Autodesk Inventor part; units mm, degrees
ref_plane "YZ Plane" through (0, 0, 0) normal (1, 0, 0) x (0, 1, 0)
ref_plane "XZ Plane" through (0, 0, 0) normal (0, 1, 0) x (-1, 0, 0)
ref_plane "XY Plane" through (0, 0, 0) normal (0, 0, 1) x (1, 0, 0)
sketch "Sketch1" plane through (0, 0, 0) normal (0, 0, 1) x (1, 0, 0)
  line L0 (-212.725, -63.5) -> (212.725, -63.5)
  line L1 (212.725, -63.5) -> (212.725, 63.5)
  line L2 (212.725, 63.5) -> (-212.725, 63.5)
  line L3 (-212.725, 63.5) -> (-212.725, -63.5)
  line L4 (-212.725, -63.5) -> (212.725, 63.5) construction
  line L5 (212.725, -63.5) -> (-212.725, 63.5) construction
  point P0 (0, 0)
  dimension "d0" = 127
  dimension "d1" = 425.45
extrude "Extrusion1" add sketch "Sketch1" along normal blind 1.5875
sketch "Sketch2" plane through (0, 0, 1.5875) normal (0, 0, 1) x (1, 0, 0)
  line L0 (152.4, -16.2954) -> (-152.4, -16.2954)
  line L1 (-152.4, -16.2954) -> (-152.4, 16.2954)
  line L2 (-152.4, 16.2954) -> (152.4, 16.2954)
  line L3 (152.4, 16.2954) -> (152.4, -16.2954)
  line L4 (152.4, -16.2954) -> (-152.4, 16.2954) construction
  line L5 (-152.4, -16.2954) -> (152.4, 16.2954) construction
  line L6 (-158.4, -5.4991) -> (-146.4, -5.4991)
  line L7 (-146.4, -5.4991) -> (-146.4, 5.4991)
  line L8 (-146.4, 5.4991) -> (-158.4, 5.4991)
  line L9 (-158.4, 5.4991) -> (-158.4, -5.4991)
  line L10 (-158.4, -5.4991) -> (-146.4, 5.4991) construction
  line L11 (-146.4, -5.4991) -> (-158.4, 5.4991) construction
  line L12 (138.9062, -15.4813) -> (165.8937, -15.4813)
  line L13 (165.8937, -15.4813) -> (165.8937, 15.4813)
  line L14 (165.8937, 15.4813) -> (138.9062, 15.4813)
  line L15 (138.9062, 15.4813) -> (138.9062, -15.4813)
  line L16 (138.9062, -15.4813) -> (165.8937, 15.4813) construction
  line L17 (165.8937, -15.4813) -> (138.9062, 15.4813) construction
  point P0 (0, 0)
  point P1 (-137.8966, 0)
  point P2 (-166.9034, 0)
  dimension "d4" = 304.8
  dimension "d5" = 12
  dimension "d6" = 10.9982
  dimension "d9" = 26.9875
  dimension "d10" = 30.9626
extrude "Extrusion2" cut sketch "Sketch2" against normal up to next contours L12 L15 L14 L3 | L3 L14 L13 L12 | L6 L9 L8 L1 | L1 L8 L7 L6
sketch "Sketch3" plane through (0, 0, 1.5875) normal (0, 0, 1) x (1, 0, 0)
  point P0 (0, 0)
hole "Hole1" at (-166.9034, 0, 1.5875) at (-137.8966, 0, 1.5875) direction (0, 0, -1) diameter 3.4036 end through all
sketch "Sketch4" plane through (0, 0, 1.5875) normal (0, 0, 1) x (1, 0, 0)
  point P0 (0, 0)
  point P1 (169.8625, 0)
  point P2 (134.9375, 0)
  point P3 (152.4, 0)
  dimension "d22" = 34.925
  dimension "d23" = 17.4625
  dimension "d24" = 152.4
hole "Hole2" at (134.9375, 0, 1.5875) at (169.8625, 0, 1.5875) direction (0, 0, -1) diameter 3.2766 end through all
properties part number "back"
Part model, mm, in its own coordinate system. Coordinates: 2 decimals unless noted, no trailing zeros. Loops run counter-clockwise (first coordinate to the right, second up) from the corner with the lowest first, then second, coordinate; pieces in that order, holes last. Notation, with made-up numbers: (86, 85) - (112, 85) arc R10 ccw to (112, 92) - close; hole circle Ø5 at (-36, 80.5). An arc over 180 degrees is marked (long way). Write each question's results on one line, items separated by ' | '. Start each with the question number.
Q1. Slice it at C-C on z = 0.5. Give the cut face in (x, y) (1 decimal).
Q2. Probe line 1 along X through (y, z) = (4, 1.15) (3 decimals); line 2 along Y through (x, z) = (158.5, 1.2); line 3 along Y through (x, z) = (-151, 0.8). List the from-to ranges inside material, lowest first.
Q3. Slice it at B-B on y = -10. Give the cut face in (x, z) (1 decimal).
Q4. Slice it at A-A on x = 154. Give the cut face in (y, z).
Answer:
1) outline: (-212.7, -63.5) - (212.7, -63.5) - (212.7, 63.5) - (-212.7, 63.5) - close; hole circle Ø3.4 at (-166.9, 0); hole (-158.4, -5.5) - (-146.4, -5.5) - (-146.4, 5.5) - (-158.4, 5.5) - close; hole circle Ø3.4 at (-137.9, 0); hole circle Ø3.3 at (134.9, 0); hole (138.9, -15.5) - (165.9, -15.5) - (165.9, 15.5) - (138.9, 15.5) - close; hole circle Ø3.3 at (169.9, 0)
2) line 1: x = -212.725 to -158.4, -146.4 to 138.906, 165.894 to 212.725 | line 2: y = -63.5 to -15.48, 15.48 to 63.5 | line 3: y = -63.5 to -5.5, 5.5 to 63.5
3) outline: (-212.7, 0) - (138.9, 0) - (138.9, 1.6) - (-212.7, 1.6) - close; (165.9, 0) - (212.7, 0) - (212.7, 1.6) - (165.9, 1.6) - close
4) outline: (-63.5, 0) - (-15.48, 0) - (-15.48, 1.59) - (-63.5, 1.59) - close; (15.48, 0) - (63.5, 0) - (63.5, 1.59) - (15.48, 1.59) - close
